Could you check a few things on this model? Use its own coordinates, in mm. A direction names the side the tool comes from. Round coordinates to 2 decimals unless told otherwise and drop trailing zeros. Loops run counter-clockwise (first coordinate to the right, second up) from the corner with the lowest first, then second, coordinate; pieces in that order, holes last. Notation, with made-up numbers: M -12.75,-21 L -6.75,-21 A10 ccw -6.75,-13 Z; hole C 28.25,80 d7. An arc over 180 degrees is marked long. One line per item, written item: value. Start each with the question number.
Q1. Which directions (+Z, -Z, +X, -X, +Y, -Y) give clear straight access to the entire face, cutting with the end or side of a thin tool? Please do faces 1 (the face through (0, 4, 0)), 2 (the face through (0, 0, -3.366)).
Q2. Imagine slicing it at B-B (z = 0). Please give me the cut outline in (x, y) (1 decimal), then the cut area to 3 significant figures.
Q3. Imagine slicing it at D-D (y = 3). Please give me the cut outline in (x, z), then the cut area to 3 significant figures.
Q4. Imagine slicing it at A-A (x = 0). Please give me the cut outline in (y, z) (1 decimal).
Q5. Please list where these lines run through material, in increasing order: line 1 along X through (y, z) = (2.25, 2.5); line 2 along X through (y, z) = (1.25, 0.5); line 3 along X through (y, z) = (3, -5).
Q6. Thinking about a two-plate mould opening in Y: for faces 3 (the face through (-5.796, 0.035, -7.559)), 4 (the face through (0, 0, 3.366)), 5 (the face through (0, -4, 0)), which applies, released by +Y, released by -Y, zero draft, split by the parting line, or undercut?
Q7. I'm going to push flat-ended pins straight in: pin 1 Ø1 at (x, y) = (-6, -0.5) entering from -Z; pin 2 Ø2 at (x, y) = (0.5, 0) entering from -Z (3 decimals); pin 3 Ø1.5 at (x, y) = (4, -2) entering from +Z; pin 4 Ø1 at (x, y) = (-4, -2) entering from +Z. Where does each tip first touch, or does it pass through?
from build123d import *

# Parameters (mm, degrees)
SKETCH1_R           = 9.525
SKETCH1_W           = 6.731
SKETCH1_H           = 6.731
BOSS_EXTRUDE1_DEPTH = 4.0005
SKETCH1_3_W         = 6.731
SKETCH1_3_H         = 6.731
CUT_EXTRUDE1_DEPTH  = 3.3655
FILLET1_R           = 1.524


with BuildPart() as part:
    # Sketch1 → Boss-Extrude1 (new, symmetric)
    with BuildSketch(Plane(origin=(0, 0, 0), x_dir=(1, 0, 0), z_dir=(0, 1, 0))):
        with Locations(Location((0, 0, 0), (0, 0, 270))):
            Circle(SKETCH1_R)
        Rectangle(SKETCH1_W, SKETCH1_H, mode=Mode.SUBTRACT)
        Rectangle(SKETCH1_W, SKETCH1_H)
    extrude(amount=BOSS_EXTRUDE1_DEPTH, both=True)

    # Sketch1_3 → Cut-Extrude1 (cut, symmetric)
    with BuildSketch(Plane(origin=(0, 0, 0), x_dir=(1, 0, 0), z_dir=(0, 1, 0))):
        Rectangle(SKETCH1_3_W, SKETCH1_3_H)
    extrude(amount=CUT_EXTRUDE1_DEPTH, both=True, mode=Mode.SUBTRACT)

    # Fillet1
    fillet1_edges = [part.edges().sort_by_distance(p)[0] for p in [
        (0, -4.0005, -9.525),
        (0, 4.0005, -9.525),
    ]]
    fillet(fillet1_edges, radius=FILLET1_R)


solid = part.part
Report:
1. face 1: +Z, -Z, +X, -X, +Y
1. face 2: none
2. outline: M -9.5,-2.5 A1.5 ccw -8,-4 L 8,-4 A1.5 ccw 9.5,-2.5 L 9.5,2.5 A1.5 ccw 8,4 L -8,4 A1.5 ccw -9.5,2.5 Z; hole M -3.4,-3.4 L 3.4,-3.4 L 3.4,3.4 L -3.4,3.4 Z
2. area: 105 mm²
3. outline: C 0,0 d18.86; hole M -3.37,-3.37 L 3.37,-3.37 L 3.37,3.37 L -3.37,3.37 Z
3. area: 234 mm²
4. outline: M -4,-8 A1.5 ccw -2.5,-9.5 L 2.5,-9.5 A1.5 ccw 4,-8 L 4,8 A1.5 ccw 2.5,9.5 L -2.5,9.5 A1.5 ccw -4,8 Z; hole M -3.4,-3.4 L 3.4,-3.4 L 3.4,3.4 L -3.4,3.4 Z
5. line 1: x = -9.19 to -3.37, 3.37 to 9.19
5. line 2: x = -9.51 to -3.37, 3.37 to 9.51
5. line 3: x = -8 to 8
6. face 3: zero draft
6. face 4: undercut
6. face 5: released by -Y
7. pin 1: stops at z = -7.78
7. pin 2: stops at z = -9.525
7. pin 3: stops at z = 8.95
7. pin 4: stops at z = 8.86
